Model file for the job. Use its own axes, mm. Face numbers are marked on the shaded views. A direction names the side the tool comes from. Give positions to 0.01 mm unless a question says otherwise; leave off trailing zeros. Order: outer loops, then holes, each group sorted by start corner. A loop starts at its lowest first (then second) coordinate and runs counter-clockwise, first axis right, second up. Notation, with made-up numbers: M 31.5,-29 L 78.5,-29 A10 cw 78.5,-20 Z; hole C -34.5,31.25 d1. An arc over 180 degrees is marked long. Return JSON: item names as keys, results as strings. Group by question number.
1. Slice it at D-D on y = -4.5. List the corners of the cut face in (x, z), then the cut area to 3 significant figures.
2. Pin check, flat tip, straight feed: pin 1 (10.5 mm diameter, centred on y = -3, z = 14, fed in from +X). Stop position of the tip, or through.
3. Slice it at A-A on z = 13.5. List the corners of the cut face in (x, y).
4. Slice it at B-B on x = 0. List the corners of the cut face in (y, z), then the cut area to 3 significant figures.
5. 3-axis set-ups, long thin cutter, end or side, ignore diameter. For the marked faces 1 and 2: which of +Z, -Z, +X, -X, +Y, -Y reach the whole face in a straight line?
6. Two-plate mould, pull along X, no slides. Class the marked faces 3, 4, 5 and 6: released by +X, released by -X, zero draft, split by the parting line, or undercut.
7. Slice it at C-C on y = 0. List the corners of the cut face in (x, z), then the cut area to 3 significant figures.
8. Wall check: probe 1 along Z at (x, y) = (-16, 0); probe 2 along Y at (x, z) = (-6, 10); probe 3 along X at (y, z) = (-10.75, 13.5). Give the ranges that are in metal, low to high. Write a range as [from, to].
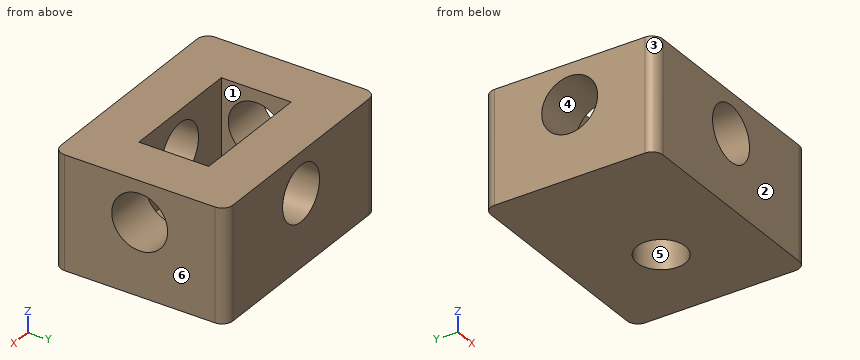
from build123d import *

# Parameters (mm, degrees)
SKETCH1_W               = 42
SKETCH1_H               = 32
BOSS_EXTRUDE1_DEPTH     = 21
SKETCH2_W               = 23
SKETCH2_H               = 13
CUT_EXTRUDE1_DEPTH      = 15
SKETCH3_R               = 4.5
CUT_EXTRUDE2_DEPTH      = 31.364452901
CUT_EXTRUDE3_DEPTH      = 42.871828238
CUT_EXTRUDE3_DEPTH_BACK = 42.871828238
SKETCH4_R               = 5.2
CUT_EXTRUDE4_DEPTH      = 38.259227045
CUT_EXTRUDE4_DEPTH_BACK = 38.259227045
SKETCH5_R               = 5.15
FILLET1_R               = 2


with BuildPart() as part:
    # Sketch1 → Boss-Extrude1 (new body)
    with BuildSketch(Plane.XY):
        Rectangle(SKETCH1_W, SKETCH1_H)
    extrude(amount=BOSS_EXTRUDE1_DEPTH)

    # Sketch2 → Cut-Extrude1 (cut)
    with BuildSketch(Plane.XY.offset(21)):
        Rectangle(SKETCH2_W, SKETCH2_H)
    extrude(amount=-CUT_EXTRUDE1_DEPTH, mode=Mode.SUBTRACT)

    # Sketch3 → Cut-Extrude2 (cut, through all)
    with BuildSketch(Plane.XY.offset(6)):
        with Locations((5.510924595, 0.660459353)):
            Circle(SKETCH3_R)
    extrude(amount=-CUT_EXTRUDE2_DEPTH, mode=Mode.SUBTRACT)

    # Sketch4 → Cut-Extrude3 (cut, two sides: drawn at the far end of the back side and taken through both)
    with BuildSketch(Plane.ZY.offset(-11.5).offset(-CUT_EXTRUDE3_DEPTH_BACK)):
        with Locations((13.5, 0)):
            Circle(SKETCH4_R)
    extrude(amount=CUT_EXTRUDE3_DEPTH + CUT_EXTRUDE3_DEPTH_BACK, mode=Mode.SUBTRACT)

    # Sketch5 → Cut-Extrude4 (cut, two sides: drawn at the far end of the back side and taken through both)
    with BuildSketch(Plane(origin=(0, -6.5, 0), x_dir=(1, 0, 0), z_dir=(0, 1, 0)).offset(-CUT_EXTRUDE4_DEPTH_BACK)):
        with Locations(Location((0, -13.5, 0), (0, 0, 180))):
            Circle(SKETCH5_R)
    extrude(amount=CUT_EXTRUDE4_DEPTH + CUT_EXTRUDE4_DEPTH_BACK, mode=Mode.SUBTRACT)

    # Fillet1
    fillet1_edges = [part.edges().sort_by_distance(p)[0] for p in [
        (-21, 16, 10.5),
        (21, 16, 10.5),
        (21, -16, 10.5),
        (-21, -16, 10.5),
    ]]
    fillet(fillet1_edges, radius=FILLET1_R)


solid = part.part
Result:
{
 "1": {"outline": "M -21,0 L 21,0 L 21,10.89 L 11.5,10.89 L 11.5,6 L -11.5,6 L -11.5,10.89 L -21,10.89 Z; M -21,16.11 L -11.5,16.11 L -11.5,21 L -21,21 Z; M 11.5,16.11 L 21,16.11 L 21,21 L 11.5,21 Z", "area": "438 mm2"},
 "2": {"pin 1": "stops at x = 21"},
 "3": {"outline": "M -21,-14 A2 ccw -19,-16 L -5.15,-16 L -5.15,-6.5 L -11.5,-6.5 L -11.5,-5.2 L -21,-5.2 Z; M -21,5.2 L -11.5,5.2 L -11.5,6.5 L -5.15,6.5 L -5.15,16 L -19,16 A2 ccw -21,14 Z; M 5.15,-16 L 19,-16 A2 ccw 21,-14 L 21,-5.2 L 11.5,-5.2 L 11.5,-6.5 L 5.15,-6.5 Z; M 5.15,6.5 L 11.5,6.5 L 11.5,5.2 L 21,5.2 L 21,14 A2 ccw 19,16 L 5.15,16 Z"},
 "4": {"outline": "M -16,0 L 16,0 L 16,8.35 L 6.5,8.35 L 6.5,6 L -6.5,6 L -6.5,8.35 L -16,8.35 Z; M -16,18.65 L -6.5,18.65 L -6.5,21 L -16,21 Z; M 6.5,18.65 L 16,18.65 L 16,21 L 6.5,21 Z", "area": "281 mm2"},
 "5": {"face 1": "+Z", "face 2": "+Z, -Z, +X, -X, -Y"},
 "6": {"face 3": "released by -X", "face 4": "zero draft", "face 5": "undercut", "face 6": "released by +X"},
 "7": {"outline": "M -21,0 L 1.06,0 L 1.06,6 L -11.5,6 L -11.5,8.3 L -21,8.3 Z; M -21,18.7 L -11.5,18.7 L -11.5,21 L -21,21 Z; M 9.96,0 L 21,0 L 21,8.3 L 11.5,8.3 L 11.5,6 L 9.96,6 Z; M 11.5,18.7 L 21,18.7 L 21,21 L 11.5,21 Z", "area": "286 mm2"},
 "8": {"probe 1": "z = [0, 8.3], [18.7, 21]", "probe 2": "y = [-16, -6.5], [6.5, 16]", "probe 3": "x = [-21, -5.15], [5.15, 21]"}
}
